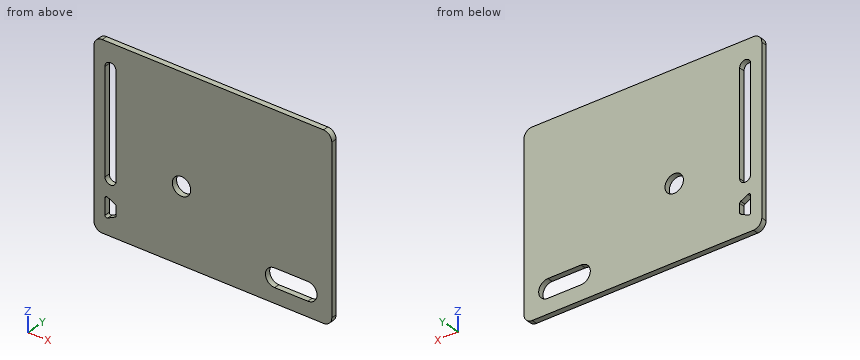
from build123d import *

# Parameters (mm, degrees)
SKETCH1_W           = 819.15
SKETCH1_H           = 622.3
BOSS_EXTRUDE1_DEPTH = 19.05
FILLET1_R           = 28.575
SKETCH2_R           = 31.75
CUT_EXTRUDE1_DEPTH  = 515.712449456
CUT_EXTRUDE2_DEPTH  = 515.712449456
CUT_EXTRUDE3_DEPTH  = 515.712449456
FILLET2_R           = 6.35
CUT_EXTRUDE4_DEPTH  = 515.712449456


with BuildPart() as part:
    # Sketch1 → Boss-Extrude1 (new body)
    with BuildSketch(Plane(origin=(0, 0, 0), x_dir=(1, 0, 0), z_dir=(0, 1, 0))):
        Rectangle(SKETCH1_W, SKETCH1_H)
    extrude(amount=BOSS_EXTRUDE1_DEPTH)

    # Fillet1
    fillet1_edges = [part.edges().sort_by_distance(p)[0] for p in [
        (409.575, 9.525, 311.15),
        (-409.575, 9.525, 311.15),
        (-409.575, 9.525, -311.15),
        (409.575, 9.525, -311.15),
    ]]
    fillet(fillet1_edges, radius=FILLET1_R)

    # Sketch2 → Cut-Extrude1 (cut, through all)
    with BuildSketch(Plane(origin=(0, 19.05, 0), x_dir=(1, 0, 0), z_dir=(0, 1, 0))):
        with Locations(Location((-107.95, 57.15, 0), (0, 0, 270))):
            Circle(SKETCH2_R)
    extrude(amount=-CUT_EXTRUDE1_DEPTH, mode=Mode.SUBTRACT)

    # Sketch3 → Cut-Extrude2 (cut, through all)
    with BuildSketch(Plane(origin=(0, 19.05, 0), x_dir=(1, 0, 0), z_dir=(0, 1, 0))):
        with BuildLine():
            Line((-333.375, 127), (-333.375, -228.6))
            ThreePointArc((-333.375, -228.6), (-352.425, -247.65), (-371.475, -228.6))
            Line((-371.475, -228.6), (-371.475, 127))
            ThreePointArc((-371.475, 127), (-352.425, 146.05), (-333.375, 127))
        make_face()
    extrude(amount=-CUT_EXTRUDE2_DEPTH, mode=Mode.SUBTRACT)

    # Sketch4 → Cut-Extrude3 (cut, through all)
    with BuildSketch(Plane(origin=(0, 19.05, 0), x_dir=(1, 0, 0), z_dir=(0, 1, 0))):
        Polygon((-371.475, 260.35), (-371.475, 184.15), (-333.375, 203.2), (-333.375, 241.3), align=None)
    extrude(amount=-CUT_EXTRUDE3_DEPTH, mode=Mode.SUBTRACT)

    # Fillet2
    fillet2_edges = [part.edges().sort_by_distance(p)[0] for p in [
        (-371.475, 9.525, -260.35),
        (-333.375, 9.525, -241.3),
        (-333.375, 9.525, -203.2),
        (-371.475, 9.525, -184.15),
    ]]
    fillet(fillet2_edges, radius=FILLET2_R)

    # Sketch5 → Cut-Extrude4 (cut, through all)
    with BuildSketch(Plane(origin=(0, 19.05, 0), x_dir=(1, 0, 0), z_dir=(0, 1, 0))):
        with BuildLine():
            Line((327.025, 196.85), (212.725, 196.85))
            ThreePointArc((212.725, 196.85), (180.975, 228.6), (212.725, 260.35))
            Line((212.725, 260.35), (327.025, 260.35))
            ThreePointArc((327.025, 260.35), (358.775, 228.6), (327.025, 196.85))
        make_face()
    extrude(amount=-CUT_EXTRUDE4_DEPTH, mode=Mode.SUBTRACT)


solid = part.part
Source: CAD feature listing. Evaluate the final solid. Frame: model axes, mm. Give positions to 0.01 mm unless a question says otherwise; leave off trailing zeros. Write each loop counter-clockwise with the first axis right and the second up, starting at its lowest first coordinate (ties: lowest second). Pieces come first, ordered by that corner, then holes. Notation, with made-up numbers: M 76.25,26 L 131.25,26 A21 ccw 131.25,39 Z; hole C 75,-26 d4. An arc over 180 degrees is marked long. Return JSON: item names as keys, results as strings. Group by question number.
1) Cut plane A-A, the plane z = 212. Output: boundary loops of the cut face in (x, y) (3 decimals), plus the area to 3 significant figures.
2) Cut plane C-C, the plane z = -228.6. Output: boundary loops of the cut face in (x, y) (3 decimals), plus the area to 3 significant figures.
3) Cut plane B-B, the plane x = -107.95. Output: boundary loops of the cut face in (y, z).
4) Material intervals for line 1 along X through (y, z) = (6.5, -57.15) (3 decimals); line 2 along X through (y, z) = (2.25, 116.5) (3 decimals); line 3 along Z through (x, y) = (-353.5, 16.75), sorted ascending. Write a range as [from, to].
5) Cut plane D-D, the plane y = 12.25. Output: boundary loops of the cut face in (x, z) (3 decimals).
Recorded:
{
 "1": {"outline": "M -409.575,0 L -371.475,0 L -371.475,19.05 L -409.575,19.05 Z; M -333.375,0 L 409.575,0 L 409.575,19.05 L -333.375,19.05 Z", "area": "14,900 mm²"},
 "2": {"outline": "M -409.575,0 L -371.475,0 L -371.475,19.05 L -409.575,19.05 Z; M -333.375,0 L 180.975,0 L 180.975,19.05 L -333.375,19.05 Z; M 358.775,0 L 409.575,0 L 409.575,19.05 L 358.775,19.05 Z", "area": "11,500 mm²"},
 "3": {"outline": "M 0,-311.15 L 19.05,-311.15 L 19.05,-88.9 L 0,-88.9 Z; M 0,-25.4 L 19.05,-25.4 L 19.05,311.15 L 0,311.15 Z"},
 "4": {"line 1": "x = [-409.575, -371.475], [-333.375, -139.7], [-76.2, 409.575]", "line 2": "x = [-409.575, -371.475], [-333.375, 409.575]", "line 3": "z = [-311.15, -251.36], [-193.14, -146.02], [247.62, 311.15]"},
 "5": {"outline": "M -409.575,-282.575 A28.575 ccw -381,-311.15 L 381,-311.15 A28.575 ccw 409.575,-282.575 L 409.575,282.575 A28.575 ccw 381,311.15 L -381,311.15 A28.575 ccw -409.575,282.575 Z; hole M -371.475,-250.075 A6.35 ccw -362.285,-255.755 L -336.885,-243.055 A6.35 ccw -333.375,-237.375 L -333.375,-207.125 A6.35 ccw -336.885,-201.445 L -362.285,-188.745 A6.35 ccw -371.475,-194.425 Z; hole M -371.475,-127 A19.05 ccw -333.375,-127 L -333.375,228.6 A19.05 ccw -371.475,228.6 Z; hole C -107.95,-57.15 d63.5; hole M 212.725,-260.35 L 327.025,-260.35 A31.75 ccw 327.025,-196.85 L 212.725,-196.85 A31.75 ccw Z"}
}
